Here's how the part is built. I have some questions about the finished solid (model axes, mm). Round coordinates to 2 decimals unless told otherwise and drop trailing zeros. Loops run counter-clockwise (first coordinate to the right, second up) from the corner with the lowest first, then second, coordinate; pieces in that order, holes last. Notation, with made-up numbers: (73.5, -15) -> (87.5, -15) arc R28 cw to (87.5, 4) -> close; hole circle Ø6 at (-21, -7). An arc over 180 degrees is marked (long way). One line per item, written item: value. Start each with the question number.
```python
from build123d import *

# Parameters (mm, degrees)
CROQUIS1_R                   = 6.5
CROQUIS1_R_2                 = 5
SALIENTE_EXTRUIR1_DEPTH      = 25
CROQUIS3_R                   = 0.5
SALIENTE_EXTRUIR2_REACH      = 32.125
SALIENTE_EXTRUIR2_END_RADIUS = 0.5
CROQUIS4_W                   = 0.5
CROQUIS4_H                   = 0.5
SALIENTE_EXTRUIR3_REACH      = 32.125
SALIENTE_EXTRUIR3_END_RADIUS = 0.5
CROQUIS6_W                   = 0.5
CROQUIS6_H                   = 0.5
CROQUIS9_R                   = 1
SALIENTE_EXTRUIR4_DEPTH      = 0.5
SIMETR_A2_COPY_1_SKETCH_R    = 1
SIMETR_A2_COPY_1_DEPTH       = 0.5
SIMETR_A3_COPY_1_SKETCH_R    = 1
SIMETR_A3_COPY_1_DEPTH       = 0.5
SIMETR_A3_COPY_2_SKETCH_R    = 1
SIMETR_A3_COPY_2_DEPTH       = 0.5
SIMETR_A3_COPY_3_SKETCH_R    = 1
SIMETR_A3_COPY_3_DEPTH       = 0.5
SIMETR_A4_COPY_1_SKETCH_R    = 1
SIMETR_A4_COPY_1_DEPTH       = 0.5
SIMETR_A4_COPY_2_SKETCH_R    = 1
SIMETR_A4_COPY_2_DEPTH       = 0.5
SIMETR_A4_COPY_3_SKETCH_R    = 1
SIMETR_A4_COPY_3_DEPTH       = 0.5
SIMETR_A4_COPY_4_SKETCH_R    = 1
SIMETR_A4_COPY_4_DEPTH       = 0.5
SIMETR_A4_COPY_5_SKETCH_R    = 1
SIMETR_A4_COPY_5_DEPTH       = 0.5
SIMETR_A4_COPY_6_SKETCH_R    = 1
SIMETR_A4_COPY_6_DEPTH       = 0.5
SIMETR_A4_COPY_7_SKETCH_R    = 1
SIMETR_A4_COPY_7_DEPTH       = 0.5
SIMETR_A4_COPY_8_SKETCH_R    = 1
SIMETR_A4_COPY_8_DEPTH       = 0.5
SIMETR_A5_COPY_1_SKETCH_R    = 1
SIMETR_A5_COPY_1_DEPTH       = 0.5
SIMETR_A5_COPY_2_SKETCH_R    = 1
SIMETR_A5_COPY_2_DEPTH       = 0.5
SIMETR_A5_COPY_3_SKETCH_R    = 1
SIMETR_A5_COPY_3_DEPTH       = 0.5
SIMETR_A5_COPY_4_SKETCH_R    = 1
SIMETR_A5_COPY_4_DEPTH       = 0.5
SIMETR_A5_COPY_5_SKETCH_R    = 1
SIMETR_A5_COPY_5_DEPTH       = 0.5
SIMETR_A5_COPY_6_SKETCH_R    = 1
SIMETR_A5_COPY_6_DEPTH       = 0.5
SIMETR_A5_COPY_7_SKETCH_R    = 1
SIMETR_A5_COPY_7_DEPTH       = 0.5
SIMETR_A5_COPY_8_SKETCH_R    = 1
SIMETR_A5_COPY_8_DEPTH       = 0.5
SIMETR_A5_COPY_9_SKETCH_R    = 1
SIMETR_A5_COPY_9_DEPTH       = 0.5


with BuildPart() as part:
    # Croquis1 → Saliente-Extruir1 (new body)
    with BuildSketch(Plane(origin=(0, 0, 0), x_dir=(1, 0, 0), z_dir=(0, 1, 0))):
        with Locations(Location((0, 0, 0), (0, 0, 270))):
            Circle(CROQUIS1_R)
        with Locations(Location((0, 0, 0), (0, 0, 270))):
            Circle(CROQUIS1_R_2, mode=Mode.SUBTRACT)
    extrude(amount=SALIENTE_EXTRUIR1_DEPTH)



with BuildPart() as body_2:
    # Barrer1: sweep along a path in Croquis2
    with BuildLine(Plane(origin=(0, 15, 0), x_dir=(1, 0, 0), z_dir=(0, 1, 0))) as barrer1_path:
        Line((-4.531635979, -6.78207252), (-1.591298939, -8))
        Line((-1.591298939, -8), (1.591298939, -8))
        Line((1.591298939, -8), (4.531635979, -6.78207252))
        Line((4.531635979, -6.78207252), (6.78207252, -4.531635979))
        Line((6.78207252, -4.531635979), (8, -1.591298939))
        Line((8, -1.591298939), (8, 1.591298939))
        Line((8, 1.591298939), (6.78207252, 4.531635979))
        Line((6.78207252, 4.531635979), (4.531635979, 6.78207252))
        Line((4.531635979, 6.78207252), (1.591298939, 8))
        Line((1.591298939, 8), (-1.591298939, 8))
        Line((-1.591298939, 8), (-4.531635979, 6.78207252))
        Line((-4.531635979, 6.78207252), (-6.78207252, 4.531635979))
        Line((-6.78207252, 4.531635979), (-8, 1.591298939))
        Line((-8, 1.591298939), (-8, -1.591298939))
        Line((-8, -1.591298939), (-6.78207252, -4.531635979))
        Line((-6.78207252, -4.531635979), (-4.531635979, -6.78207252))
    # Croquis3 → Barrer1 (sweep)
    with BuildSketch(Plane(origin=(0, 0, 0), x_dir=(0, 0, -1), z_dir=(1, 0, 0))):
        with Locations((-8, 15)):
            Circle(CROQUIS3_R)
    sweep(path=barrer1_path.line, transition=Transition.RIGHT)


with BuildPart() as part_1:
    add(part.part)

    add(body_2.part)  # Saliente-Extruir2 merges body 2
    # Saliente-Extruir2: up to this cylinder (the profile starts outside it)
    saliente_extruir2_end = Plane(origin=(0, 15, 8), z_dir=(-1, 0, 0)) * Cylinder(SALIENTE_EXTRUIR2_END_RADIUS, 66.25, mode=Mode.PRIVATE)
    # Croquis4 → Saliente-Extruir2 (add, up to the surface)
    with BuildSketch(Plane.XY.offset(6), mode=Mode.PRIVATE) as saliente_extruir2_sk1:
        with Locations((0, 15)):
            Rectangle(CROQUIS4_W, CROQUIS4_H)
    saliente_extruir2_tool1 = extrude(saliente_extruir2_sk1.sketch, amount=SALIENTE_EXTRUIR2_REACH, mode=Mode.PRIVATE) - saliente_extruir2_end
    add(saliente_extruir2_tool1.solids().sort_by_distance((0, 15, 6))[0])

    # Saliente-Extruir3: up to this cylinder (the profile starts outside it)
    saliente_extruir3_end = Plane(origin=(0, 15, -8), z_dir=(1, 0, 0)) * Cylinder(SALIENTE_EXTRUIR3_END_RADIUS, 66.25, mode=Mode.PRIVATE)
    # Croquis6 → Saliente-Extruir3 (add, up to the surface)
    with BuildSketch(Plane.XY.offset(-6), mode=Mode.PRIVATE) as saliente_extruir3_sk1:
        with Locations((0, 15)):
            Rectangle(CROQUIS6_W, CROQUIS6_H)
    saliente_extruir3_tool1 = extrude(saliente_extruir3_sk1.sketch, amount=-SALIENTE_EXTRUIR3_REACH, mode=Mode.PRIVATE) - saliente_extruir3_end
    add(saliente_extruir3_tool1.solids().sort_by_distance((0, 15, -6))[0])

    # Croquis9 → Saliente-Extruir4 (add)
    with BuildSketch(Plane(origin=(-0.461939766, 0, -0.191341716), x_dir=(-0.3826834323650839, 0, 0.9238795325112892), z_dir=(-0.9238795325112892, 0, -0.3826834323650839))):
        with Locations((8, 15)):
            Circle(CROQUIS9_R)
    saliente_extruir4 = extrude(amount=SALIENTE_EXTRUIR4_DEPTH)

    # Simetría1: Saliente-Extruir4 across plane
    add(saliente_extruir4.mirror(Plane(origin=(0, 0, 0), x_dir=(-0.3826834323650839, 0, 0.9238795325112891), z_dir=(-0.9238795325112892, 0, -0.3826834323650839))))

    # Simetría2: Saliente-Extruir4 across plane
    add(saliente_extruir4.mirror(Plane.XY))

    # Simetría2 copy 1 sketch → Simetría2 copy 1 (add)
    with BuildSketch(Plane(origin=(0.461939766, 0, -0.191341716), x_dir=(-0.38268343236508395, 0, -0.9238795325112892), z_dir=(0.9238795325112892, 0, -0.38268343236508395))):
        with Locations((8, 15)):
            Circle(SIMETR_A2_COPY_1_SKETCH_R)
    extrude(amount=SIMETR_A2_COPY_1_DEPTH)

    # Simetría3: Saliente-Extruir4 across plane
    add(saliente_extruir4.mirror(Plane(origin=(0, 0, 0), x_dir=(0, 0, 1), z_dir=(1, 0, 0))))

    # Simetría3 copy 1 sketch → Simetría3 copy 1 (add)
    with BuildSketch(Plane(origin=(-0.461939766, 0, 0.191341716), x_dir=(0.38268343236508395, 0, 0.9238795325112892), z_dir=(-0.9238795325112892, 0, 0.38268343236508395))):
        with Locations((8, 15)):
            Circle(SIMETR_A3_COPY_1_SKETCH_R)
    extrude(amount=SIMETR_A3_COPY_1_DEPTH)

    # Simetría3 copy 2 sketch → Simetría3 copy 2 (add)
    with BuildSketch(Plane(origin=(0.461939766, 0, 0.191341716), x_dir=(0.3826834323650839, 0, -0.9238795325112892), z_dir=(0.9238795325112892, 0, 0.3826834323650839))):
        with Locations((8, 15)):
            Circle(SIMETR_A3_COPY_2_SKETCH_R)
    extrude(amount=SIMETR_A3_COPY_2_DEPTH)

    # Simetría3 copy 3 sketch → Simetría3 copy 3 (add)
    with BuildSketch(Plane(origin=(-0.461939766, 0, -0.191341716), x_dir=(0.38268343236508395, 0, -0.9238795325112892), z_dir=(-0.9238795325112892, 0, -0.38268343236508395))):
        with Locations((8, -15)):
            Circle(SIMETR_A3_COPY_3_SKETCH_R)
    extrude(amount=SIMETR_A3_COPY_3_DEPTH)

    # Simetría4 copy 1 sketch → Simetría4 copy 1 (add)
    with BuildSketch(Plane(origin=(0.191341716, 0, 0.461939766), x_dir=(0.9238795325112795, 0, -0.3826834323651074), z_dir=(0.3826834323651074, 0, 0.9238795325112795))):
        with Locations((8, 15)):
            Circle(SIMETR_A4_COPY_1_SKETCH_R)
    extrude(amount=SIMETR_A4_COPY_1_DEPTH)

    # Simetría4 copy 2 sketch → Simetría4 copy 2 (add)
    with BuildSketch(Plane(origin=(-0.191341716, 0, -0.461939766), x_dir=(0.9238795325112796, 0, -0.3826834323651075), z_dir=(-0.3826834323651075, 0, -0.9238795325112796))):
        with Locations((8, -15)):
            Circle(SIMETR_A4_COPY_2_SKETCH_R)
    extrude(amount=SIMETR_A4_COPY_2_DEPTH)

    # Simetría4 copy 3 sketch → Simetría4 copy 3 (add)
    with BuildSketch(Plane(origin=(0.461939766, 0, 0.191341716), x_dir=(-0.38268343236508395, 0, 0.9238795325112892), z_dir=(0.9238795325112892, 0, 0.38268343236508395))):
        with Locations((8, -15)):
            Circle(SIMETR_A4_COPY_3_SKETCH_R)
    extrude(amount=SIMETR_A4_COPY_3_DEPTH)

    # Simetría4 copy 4 sketch → Simetría4 copy 4 (add)
    with BuildSketch(Plane(origin=(-0.191341716, 0, -0.461939766), x_dir=(-0.9238795325112795, 0, 0.3826834323651074), z_dir=(-0.3826834323651074, 0, -0.9238795325112795))):
        with Locations((8, 15)):
            Circle(SIMETR_A4_COPY_4_SKETCH_R)
    extrude(amount=SIMETR_A4_COPY_4_DEPTH)

    # Simetría4 copy 5 sketch → Simetría4 copy 5 (add)
    with BuildSketch(Plane(origin=(0.191341716, 0, 0.461939766), x_dir=(-0.9238795325112796, 0, 0.3826834323651075), z_dir=(0.3826834323651075, 0, 0.9238795325112796))):
        with Locations((8, -15)):
            Circle(SIMETR_A4_COPY_5_SKETCH_R)
    extrude(amount=SIMETR_A4_COPY_5_DEPTH)

    # Simetría4 copy 6 sketch → Simetría4 copy 6 (add)
    with BuildSketch(Plane(origin=(-0.461939766, 0, -0.191341716), x_dir=(0.38268343236508395, 0, -0.9238795325112892), z_dir=(-0.9238795325112892, 0, -0.38268343236508395))):
        with Locations((8, -15)):
            Circle(SIMETR_A4_COPY_6_SKETCH_R)
    extrude(amount=SIMETR_A4_COPY_6_DEPTH)

    # Simetría4 copy 7 sketch → Simetría4 copy 7 (add)
    with BuildSketch(Plane(origin=(0.461939766, 0, 0.191341716), x_dir=(0.3826834323650839, 0, -0.9238795325112892), z_dir=(0.9238795325112892, 0, 0.3826834323650839))):
        with Locations((8, 15)):
            Circle(SIMETR_A4_COPY_7_SKETCH_R)
    extrude(amount=SIMETR_A4_COPY_7_DEPTH)

    # Simetría4 copy 8 sketch → Simetría4 copy 8 (add)
    with BuildSketch(Plane(origin=(0.461939766, 0, 0.191341716), x_dir=(-0.38268343236508395, 0, 0.9238795325112892), z_dir=(0.9238795325112892, 0, 0.38268343236508395))):
        with Locations((8, -15)):
            Circle(SIMETR_A4_COPY_8_SKETCH_R)
    extrude(amount=SIMETR_A4_COPY_8_DEPTH)

    # Simetría5 copy 1 sketch → Simetría5 copy 1 (add)
    with BuildSketch(Plane(origin=(-0.191341716, 0, 0.461939766), x_dir=(-0.9238795325112795, 0, -0.3826834323651074), z_dir=(-0.3826834323651074, 0, 0.9238795325112795))):
        with Locations((8, -15)):
            Circle(SIMETR_A5_COPY_1_SKETCH_R)
    extrude(amount=SIMETR_A5_COPY_1_DEPTH)

    # Simetría5 copy 2 sketch → Simetría5 copy 2 (add)
    with BuildSketch(Plane(origin=(0.191341716, 0, -0.461939766), x_dir=(-0.9238795325112796, 0, -0.3826834323651075), z_dir=(0.3826834323651075, 0, -0.9238795325112796))):
        with Locations((8, 15)):
            Circle(SIMETR_A5_COPY_2_SKETCH_R)
    extrude(amount=SIMETR_A5_COPY_2_DEPTH)

    # Simetría5 copy 3 sketch → Simetría5 copy 3 (add)
    with BuildSketch(Plane(origin=(-0.461939766, 0, 0.191341716), x_dir=(0.38268343236508395, 0, 0.9238795325112892), z_dir=(-0.9238795325112892, 0, 0.38268343236508395))):
        with Locations((8, 15)):
            Circle(SIMETR_A5_COPY_3_SKETCH_R)
    extrude(amount=SIMETR_A5_COPY_3_DEPTH)

    # Simetría5 copy 4 sketch → Simetría5 copy 4 (add)
    with BuildSketch(Plane(origin=(0.191341716, 0, -0.461939766), x_dir=(0.9238795325112795, 0, 0.3826834323651074), z_dir=(0.3826834323651074, 0, -0.9238795325112795))):
        with Locations((8, -15)):
            Circle(SIMETR_A5_COPY_4_SKETCH_R)
    extrude(amount=SIMETR_A5_COPY_4_DEPTH)

    # Simetría5 copy 5 sketch → Simetría5 copy 5 (add)
    with BuildSketch(Plane(origin=(-0.191341716, 0, 0.461939766), x_dir=(0.9238795325112796, 0, 0.3826834323651075), z_dir=(-0.3826834323651075, 0, 0.9238795325112796))):
        with Locations((8, 15)):
            Circle(SIMETR_A5_COPY_5_SKETCH_R)
    extrude(amount=SIMETR_A5_COPY_5_DEPTH)

    # Simetría5 copy 6 sketch → Simetría5 copy 6 (add)
    with BuildSketch(Plane(origin=(0.461939766, 0, -0.191341716), x_dir=(-0.38268343236508395, 0, -0.9238795325112892), z_dir=(0.9238795325112892, 0, -0.38268343236508395))):
        with Locations((8, 15)):
            Circle(SIMETR_A5_COPY_6_SKETCH_R)
    extrude(amount=SIMETR_A5_COPY_6_DEPTH)

    # Simetría5 copy 7 sketch → Simetría5 copy 7 (add)
    with BuildSketch(Plane(origin=(-0.461939766, 0, 0.191341716), x_dir=(-0.3826834323650839, 0, -0.9238795325112892), z_dir=(-0.9238795325112892, 0, 0.3826834323650839))):
        with Locations((8, -15)):
            Circle(SIMETR_A5_COPY_7_SKETCH_R)
    extrude(amount=SIMETR_A5_COPY_7_DEPTH)

    # Simetría5 copy 8 sketch → Simetría5 copy 8 (add)
    with BuildSketch(Plane(origin=(-0.461939766, 0, 0.191341716), x_dir=(0.38268343236508395, 0, 0.9238795325112892), z_dir=(-0.9238795325112892, 0, 0.38268343236508395))):
        with Locations((8, 15)):
            Circle(SIMETR_A5_COPY_8_SKETCH_R)
    extrude(amount=SIMETR_A5_COPY_8_DEPTH)

    # Simetría5 copy 9 sketch → Simetría5 copy 9 (add)
    with BuildSketch(Plane(origin=(0.461939766, 0, -0.191341716), x_dir=(0.3826834323650839, 0, 0.9238795325112892), z_dir=(0.9238795325112892, 0, -0.3826834323650839))):
        with Locations((8, -15)):
            Circle(SIMETR_A5_COPY_9_SKETCH_R)
    extrude(amount=SIMETR_A5_COPY_9_DEPTH)


solid = part_1.part
```
Q1. If I drill on line 1 along X through (y, z) = (6.25, 0); line 2 along Z through (x, y) = (4.5, 6.25); line 3 along Z through (x, y) = (2.5, 6.5), over which ranges is the centre line in solid material (lowest first)?
Q2. I want a section at B-B on y = 1.5. Please give me the cut outline in (x, z), plus the area to 3 significant figures.
Q3. I want a section at A-A on z = 0. Please give me the cut outline in (x, y), plus the area to 3 significant figures.
Q4. Will these pins go through, and if not, where does the flat tip stop? P1, Ø6, axis at x = 7, y = 13, coming from the -Z side; P2, Ø1, axis at x = 3.5, z = -2.5, coming from the +Y side; P3, Ø0.6, axis at y = 15, z = -7, coming from the -X side; P4, Ø4, axis at y = 7.5, z = 0.5, coming from the +X side.
Q5. I want a section at C-C on z = 5.5. State how many separate pieces and enclosed holes the cut face has, plus the area to 3 significant figures.
Answers below:
1. line 1: x = -6.5 to -5, 5 to 6.5
1. line 2: z = -4.69 to -2.18, 2.18 to 4.69
1. line 3: z = -6 to -4.33, 4.33 to 6
2. outline: circle Ø13 at (0, 0); hole circle Ø10 at (0, 0)
2. area: 54.2 mm^2
3. outline: circle Ø1 at (-8, 15); (-6.5, 0) -> (-5, 0) -> (-5, 25) -> (-6.5, 25) -> close; (5, 0) -> (6.5, 0) -> (6.5, 25) -> (5, 25) -> close; circle Ø1 at (8, 15)
3. area: 76.6 mm^2
4. P1: stops at z = -7.25
4. P2: passes through
4. P3: stops at x = -5.32
4. P4: stops at x = 6.5
5. separate pieces: 3
5. enclosed holes: 0
5. area: 175 mm^2
